Here's how the part is built. I have some questions about the finished solid (model axes, mm). A direction names the side the tool comes from. Round coordinates to 2 decimals unless told otherwise and drop trailing zeros. Loops run counter-clockwise (first coordinate to the right, second up) from the corner with the lowest first, then second, coordinate; pieces in that order, holes last. Notation, with made-up numbers: M 67.5,54 L 115.5,54 A28 cw 115.5,91 Z; hole C 89.25,-29 d9. An arc over 180 degrees is marked long. Write each question's results on one line, items separated by ' | '. Start each with the question number.
```python
from build123d import *

# Parameters (mm, degrees)
SKETCH_2_W          = 3
SKETCH_2_H          = 2.405661247
CUT_EXTRUDE_1_DEPTH = 19


with BuildPart() as part:
    # Эскиз1 → Повернуть1 (revolve)
    with BuildSketch(Plane(origin=(0, 0, 0), x_dir=(0, 0, -1), z_dir=(1, 0, 0))):
        with BuildLine():
            Line((15, 7), (15, 4.8))
            ThreePointArc((15, 4.8), (14.7, 4.5), (15, 4.2))
            Line((15, 4.2), (14.982695469, -4.100374484))
            ThreePointArc((14.982695469, -4.100374484), (14.600374484, -4.517304531), (15.017304531, -4.899625516))
            Line((15.017304531, -4.899625516), (15.017304531, -7))
            Line((15.017304531, -7), (10.850882415, -7))
            Line((10.850882415, -7), (8.840023423, -9))
            Line((8.840023423, -9), (5, -9))
            Line((5, -9), (5, 9))
            Line((5, 9), (8.840023423, 9))
            Line((8.840023423, 9), (10.850882415, 7))
            Line((10.850882415, 7), (15, 7))
        make_face()
    revolve(axis=Axis((0, 26.633173064, 0), (0, -1, 0)))

    # Эскиз2 → Вырез-Вытянуть1 (cut, through all)
    with BuildSketch(Plane(origin=(0, 9, 0), x_dir=(1, 0, 0), z_dir=(0, 1, 0))):
        with Locations((0, 5.202830624)):
            Rectangle(SKETCH_2_W, SKETCH_2_H)
    extrude(amount=-CUT_EXTRUDE_1_DEPTH, mode=Mode.SUBTRACT)


solid = part.part
```
Item 1: I'm going to push flat-ended pins straight in: pin 1 (6 mm diameter, centred on y = 1, z = -9.5, fed in from -X); pin 2 (4 mm diameter, centred on x = -4, y = 5, fed in from -Z); pin 3 (3.5 mm diameter, centred on x = 0.5, y = 1.5, fed in from +Z). Where does each tip first touch, or does it pass through?
Item 2: I need wall thicknesses on L1, parallel to X at y = 2.25, z = 0; L2, parallel to X at y = 2.25, z = -1.5; L3, parallel to Y at x = 13, z = -6. Which ranges of each line are inside material? Lowest first, please.
Item 3: If we section it at B-B on y = -5.75: Please give me the cut outline in (x, z).
Item 4: Which directions (+Z, -Z, +X, -X, +Y, -Y) give clear straight access to the entire face, cutting with the end or side of a thin tool? Please do faces 5 (the face through (1.5, 0, -6)), 6 (the face through (5, -7, -10)), 7 (the face through (-4, -9, -4)).
Item 5: If we mould it in two halves opening along Z, with no side actions, what happens to faces 1 (the face through (5, 7, 10)), 2 (the face through (0, 0, 5)), 3 (the face through (0.66, 5.885, 14.985)), 4 (the face through (-1.5, 0, -6))? For each: released by +Z, released by -Z, zero draft, split by the parting line, or undercut.
Item 6: If we section it at A-A on y = 5.5: Please give me the cut outline in (x, z).
Numbers:
1) pin 1: x = -13.51 | pin 2: z = -14.87 | pin 3: z = 15
2) L1: -15 to -5, 5 to 15 | L2: -14.92 to -4.77, 4.77 to 14.92 | L3: -7 to 7
3) outline: C 0,0 d30.03; hole M -1.5,-6.41 L 1.5,-6.41 L 1.5,-4.77 A5 ccw long -1.5,-4.77 Z
4) face 5: +Y, -Y | face 6: -Y | face 7: +Z, -Z, +X, -X, -Y
5) face 1: zero draft | face 2: undercut | face 3: split by the parting line | face 4: undercut
6) outline: C 0,0 d30; hole M -1.5,-6.41 L 1.5,-6.41 L 1.5,-4.77 A5 ccw long -1.5,-4.77 Z
